Source: CAD feature listing. Evaluate the final solid. Frame: model axes, mm. Face numbers are marked on the shaded views. A direction names the side the tool comes from. Coordinates: 2 decimals unless noted, no trailing zeros. Loops run counter-clockwise (first coordinate to the right, second up) from the corner with the lowest first, then second, coordinate; pieces in that order, holes last. Notation, with made-up numbers: (38, 35) -> (75, 35) arc R22 cw to (75, 69) -> close; hole circle Ø1 at (-39, -11). An arc over 180 degrees is marked (long way). Answer as a JSON object with one key per item and string values. Group by question number.
from build123d import *

# Parameters (mm, degrees)
SKETCH1_W                    = 710
SKETCH1_H                    = 500
BASE_FLANGE1_DEPTH           = 10
EDGE_FLANGE1_STRIP_W         = 41.4732
EDGE_FLANGE1_STRIP_H         = 10
EDGE_FLANGE1_STRIP_CUT_DEPTH = 500
EDGE_FLANGE1_DEPTH           = 500
EDGE_FLANGE2_STRIP_W         = 41.4732
EDGE_FLANGE2_STRIP_H         = 10
EDGE_FLANGE2_STRIP_CUT_DEPTH = 500
EDGE_FLANGE2_DEPTH           = 500
SKETCH12_R                   = 8.5
CUT_EXTRUDE1_DEPTH           = 757.967634711
LPATTERN1_COUNT              = 3
LPATTERN1_PITCH              = 190
SKETCH13_R                   = 11
CUT_EXTRUDE2_DEPTH           = 442.503114372
LPATTERN2_COUNT              = 2
LPATTERN2_PITCH              = 405
LPATTERN2_COUNT_DIR2         = 2
LPATTERN2_PITCH_DIR2         = 350


# Sheet-metal steps are written as plain solids
with BuildPart() as part:
    # Sketch1 → Base-Flange1 (new body)
    with BuildSketch(Plane.XY):
        Rectangle(SKETCH1_W, SKETCH1_H)
    extrude(amount=-BASE_FLANGE1_DEPTH)

    # Edge-Flange1 strip (across the edge) → Edge-Flange1 strip cut (cut)
    with BuildSketch(Plane(origin=(-355, -250, -10), x_dir=(1, 0, 0), z_dir=(0, 1, 0))):
        with Locations((-10, -5)):
            Rectangle(EDGE_FLANGE1_STRIP_W, EDGE_FLANGE1_STRIP_H)
    extrude(amount=EDGE_FLANGE1_STRIP_CUT_DEPTH, mode=Mode.SUBTRACT)

    # Edge-Flange1 section (across the edge) → Edge-Flange1 (add)
    with BuildSketch(Plane(origin=(-355, -250, -10), x_dir=(1, 0, 0), z_dir=(0, 1, 0))):
        with BuildLine():
            Line((0, 0.7366), (0, 70))
            Line((0, 70), (10, 70))
            Line((10, 70), (10, 0.7366))
            ThreePointArc((10, 0.7366), (10.215745145, 0.215745145), (10.7366, 0))
            Line((10.7366, 0), (10.7366, -10))
            ThreePointArc((10.7366, -10), (3.144677333, -6.855322667), (0, 0.7366))
        make_face()
    extrude(amount=EDGE_FLANGE1_DEPTH)

    # Edge-Flange2 strip (across the edge) → Edge-Flange2 strip cut (cut)
    with BuildSketch(Plane(origin=(355, 250, -10), x_dir=(-1, 0, 0), z_dir=(0, -1, 0))):
        with Locations((-10, -5)):
            Rectangle(EDGE_FLANGE2_STRIP_W, EDGE_FLANGE2_STRIP_H)
    extrude(amount=EDGE_FLANGE2_STRIP_CUT_DEPTH, mode=Mode.SUBTRACT)

    # Edge-Flange2 section (across the edge) → Edge-Flange2 (add)
    with BuildSketch(Plane(origin=(355, 250, -10), x_dir=(-1, 0, 0), z_dir=(0, -1, 0))):
        with BuildLine():
            Line((0, 0.7366), (0, 70))
            Line((0, 70), (10, 70))
            Line((10, 70), (10, 0.7366))
            ThreePointArc((10, 0.7366), (10.215745145, 0.215745145), (10.7366, 0))
            Line((10.7366, 0), (10.7366, -10))
            ThreePointArc((10.7366, -10), (3.144677333, -6.855322667), (0, 0.7366))
        make_face()
    extrude(amount=EDGE_FLANGE2_DEPTH)

    # Sketch12 → Cut-Extrude1 (cut, symmetric)
    with BuildSketch(Plane.ZY.offset(355)):
        with Locations((-40, 190)):
            Circle(SKETCH12_R)
    cut_extrude1 = extrude(amount=CUT_EXTRUDE1_DEPTH, both=True, mode=Mode.SUBTRACT)

    # LPattern1: Cut-Extrude1 ×3
    with Locations(*[(0, -i * LPATTERN1_PITCH, 0) for i in range(1, LPATTERN1_COUNT)]):
        add(cut_extrude1, mode=Mode.SUBTRACT)

    # Sketch13 → Cut-Extrude2 (cut, symmetric)
    with BuildSketch(Plane.XY):
        with Locations((202.5, 175)):
            Circle(SKETCH13_R)
    cut_extrude2 = extrude(amount=CUT_EXTRUDE2_DEPTH, both=True, mode=Mode.SUBTRACT)

    # LPattern2: Cut-Extrude2 2 × 2
    with Locations(*[(-i * LPATTERN2_PITCH, -j * LPATTERN2_PITCH_DIR2, 0) for i in range(LPATTERN2_COUNT) for j in range(LPATTERN2_COUNT_DIR2) if (i, j) != (0, 0)]):
        add(cut_extrude2, mode=Mode.SUBTRACT)


solid = part.part
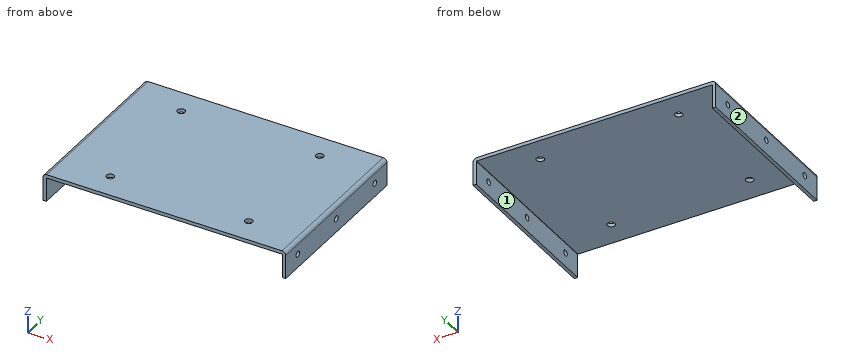
1. Reachability of the marked faces 1 and 2 from +Z, -Z, +X, -X, +Y, -Y: full face, straight path, thin tool, end or side. Return the list, or none.
2. Ray query, L1, parallel to Y at x = 347, z = -40; L2, parallel to X at y = 49.5, z = -54; L3, parallel to Y at x = -202.5, z = -3.75. Return the intervals inside material, ascending.
3. Section query A-A on z = -40. State how many separate pieces and enclosed holes the cut face has, then the cut area to 3 significant figures.
4. Section query D-D on z = -73. Return loops of the section in (x, y).
5. Pin query (flat end, axial travel): pin 1 Ø8 at (x, y) = (218, -159.5) entering from -Z. Return the tip coordinate at first contact, or that it passes through.
6. Section query B-B on x = -202.5. Return loops of the section in (y, z), then the cut area to 3 significant figures.
7. Section query C-C on y = 0. Return loops of the section in (x, z).
Solved:
{
 "1": {"face 1": "-Z, +Y, -Y", "face 2": "+Z, -Z, -X, +Y, -Y"},
 "2": {"L1": "-250 to -198.5, -181.5 to -8.5, 8.5 to 181.5, 198.5 to 250", "L2": "-355 to -345, 345 to 355", "L3": "-250 to -186, -164 to 164, 186 to 250"},
 "3": {"separate pieces": "8", "enclosed holes": "0", "area": "8,980 mm^2"},
 "4": {"outline": "(-355, -250) -> (-345, -250) -> (-345, 250) -> (-355, 250) -> close; (345, -250) -> (355, -250) -> (355, 250) -> (345, 250) -> close"},
 "5": {"pin 1": "z = -10"},
 "6": {"outline": "(-250, -10) -> (-186, -10) -> (-186, 0) -> (-250, 0) -> close; (-164, -10) -> (164, -10) -> (164, 0) -> (-164, 0) -> close; (186, -10) -> (250, -10) -> (250, 0) -> (186, 0) -> close", "area": "4,560 mm^2"},
 "7": {"outline": "(-355, -80) -> (-345, -80) -> (-345, -48.5) -> (-355, -48.5) -> close; (-355, -31.5) -> (-345, -31.5) -> (-345, -10.74) arc R0.74 cw to (-344.26, -10) -> (344.26, -10) arc R0.74 cw to (345, -10.74) -> (345, -31.5) -> (355, -31.5) -> (355, -10.74) arc R10.74 ccw to (344.26, 0) -> (-344.26, 0) arc R10.74 ccw to (-355, -10.74) -> close; (345, -80) -> (355, -80) -> (355, -48.5) -> (345, -48.5) -> close"}
}
